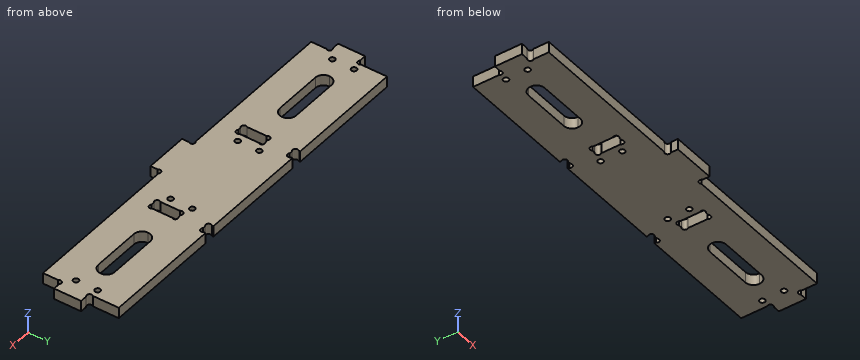
Autodesk Inventor part; units mm, degrees
ref_plane "YZ Plane" through (0, 0, 0) normal (1, 0, 0) x (0, 1, 0)
ref_plane "XZ Plane" through (0, 0, 0) normal (0, 1, 0) x (-1, 0, 0)
ref_plane "XY Plane" through (0, 0, 0) normal (0, 0, 1) x (1, 0, 0)
sketch "Sketch1" plane through (0, 0, 0) normal (0, 0, 1) x (1, 0, 0)
  line L0 (0, 0) -> (457.2, 0)
  line L1 (457.2, 0) -> (457.2, 101.6)
  line L2 (457.2, 101.6) -> (0, 101.6)
  line L3 (0, 101.6) -> (0, 0)
  line L4 (0, 101.6) -> (12.7, 101.6)
  line L5 (12.7, 101.6) -> (12.7, 66.675)
  line L6 (12.7, 66.675) -> (0, 66.675)
  line L7 (0, 66.675) -> (0, 101.6)
  line L8 (457.2, 101.6) -> (444.5, 101.6)
  line L9 (444.5, 101.6) -> (444.5, 66.675)
  line L10 (444.5, 66.675) -> (457.2, 66.675)
  line L11 (457.2, 66.675) -> (457.2, 101.6)
  line L12 (0, 0) -> (12.7, 0)
  line L13 (12.7, 0) -> (12.7, 34.925)
  line L14 (12.7, 34.925) -> (0, 34.925)
  line L15 (0, 34.925) -> (0, 0)
  line L16 (457.2, 0) -> (444.5, 0)
  line L17 (444.5, 0) -> (444.5, 34.925)
  line L18 (444.5, 34.925) -> (457.2, 34.925)
  line L19 (457.2, 34.925) -> (457.2, 0)
  line L20 (152.4, 101.6) -> (165.1, 101.6)
  line L21 (165.1, 101.6) -> (165.1, 95.25)
  line L22 (165.1, 95.25) -> (152.4, 95.25)
  line L23 (152.4, 95.25) -> (152.4, 101.6)
  line L24 (304.8, 101.6) -> (292.1, 101.6)
  line L25 (292.1, 101.6) -> (292.1, 95.25)
  line L26 (292.1, 95.25) -> (304.8, 95.25)
  line L27 (304.8, 95.25) -> (304.8, 101.6)
  line L28 (152.4, 66.675) -> (165.1, 66.675)
  line L29 (165.1, 66.675) -> (165.1, 34.925)
  line L30 (165.1, 34.925) -> (152.4, 34.925)
  line L31 (152.4, 34.925) -> (152.4, 66.675)
  line L32 (292.1, 66.675) -> (304.8, 66.675)
  line L33 (304.8, 66.675) -> (304.8, 34.925)
  line L34 (304.8, 34.925) -> (292.1, 34.925)
  line L35 (292.1, 34.925) -> (292.1, 66.675)
  line L36 (12.7, 0) -> (203.2, 0)
  line L37 (203.2, 0) -> (203.2, 12.7)
  line L38 (203.2, 12.7) -> (12.7, 12.7)
  line L39 (12.7, 12.7) -> (12.7, 0)
  line L40 (444.5, 0) -> (254, 0)
  line L41 (254, 0) -> (254, 12.7)
  line L42 (254, 12.7) -> (444.5, 12.7)
  line L43 (444.5, 12.7) -> (444.5, 0)
  point P0 (0, 66.675)
  point P1 (12.7, 12.7)
  point P2 (292.1, 101.6)
  point P3 (165.1, 101.6)
  dimension "d0" = 101.6
  dimension "d1" = 457.2
  dimension "d2" = 12.7
  dimension "d3" = 34.925
  dimension "d4" = 12.7
  dimension "d5" = 34.925
  dimension "d6" = 12.7
  dimension "d7" = 34.925
  dimension "d8" = 12.7
  dimension "d9" = 34.925
  dimension "d13" = 12.7
  dimension "d14" = 6.35
  dimension "d15" = 139.7
  dimension "d16" = 12.7
  dimension "d17" = 6.35
  dimension "d18" = 139.7
  dimension "d19" = 12.7
  dimension "d20" = 139.7
  dimension "d21" = 28.575
  dimension "d22" = 12.7
  dimension "d23" = 139.7
  dimension "d24" = 28.575
  dimension "d25" = 31.75
  dimension "d26" = 31.75
  dimension "d27" = 190.5
  dimension "d28" = 12.7
  dimension "d29" = 190.5
  dimension "d30" = 12.7
extrude "Extrusion1" add sketch "Sketch1" along normal blind 12.7 contours L3 L6 L5 L2 L23 L22 L21 L25 L26 L27 L9 L10 L1 L18 L17 L42 L41 L0 L37 L38 L13 L14
sketch "Sketch3" plane through (0, 0, 12.7) normal (0, 0, 1) x (1, 0, 0)
  line L0 (12.7, 101.6) -> (12.7, 66.675)
  line L1 (12.7, 66.675) -> (10.4549, 68.9201)
  circle A0 centre (10.4549, 68.9201) radius 3.175
  line L2 (12.7, 34.925) -> (12.7, 12.7)
  line L3 (12.7, 34.925) -> (10.4549, 32.6799)
  circle A1 centre (10.4549, 32.6799) radius 3.175
  line L4 (203.2, 12.7) -> (203.2, 0)
  line L5 (203.2, 12.7) -> (200.9549, 10.4549)
  circle A2 centre (200.9549, 10.4549) radius 3.175
  line L6 (254, 0) -> (254, 12.7)
  line L7 (254, 12.7) -> (256.2451, 10.4549)
  line L8 (254, 12.7) -> (444.5, 12.7)
  circle A3 centre (256.2451, 10.4549) radius 3.175
  line L9 (444.5, 34.925) -> (446.7451, 32.6799)
  line L10 (444.5, 34.925) -> (457.2, 34.925)
  circle A4 centre (446.7451, 32.6799) radius 3.175
  line L11 (457.2, 66.675) -> (444.5, 66.675)
  line L12 (444.5, 66.675) -> (446.7451, 68.9201)
  circle A5 centre (446.7451, 68.9201) radius 3.175
  line L13 (304.8, 34.925) -> (292.1, 34.925)
  line L14 (292.1, 34.925) -> (294.3451, 37.1701)
  line L15 (304.8, 34.925) -> (302.5549, 37.1701)
  line L16 (304.8, 66.675) -> (304.8, 34.925)
  line L17 (292.1, 66.675) -> (304.8, 66.675)
  line L18 (292.1, 66.675) -> (294.3451, 64.4299)
  line L19 (304.8, 66.675) -> (302.5549, 64.4299)
  line L20 (304.8, 95.25) -> (292.1, 95.25)
  line L21 (292.1, 95.25) -> (294.3451, 97.4951)
  line L22 (304.8, 95.25) -> (302.5549, 97.4951)
  line L23 (304.8, 101.6) -> (304.8, 95.25)
  line L24 (165.1, 34.925) -> (152.4, 34.925)
  line L25 (152.4, 34.925) -> (154.6451, 37.1701)
  line L26 (165.1, 66.675) -> (165.1, 34.925)
  line L27 (165.1, 34.925) -> (162.8549, 37.1701)
  line L28 (152.4, 66.675) -> (165.1, 66.675)
  line L29 (152.4, 66.675) -> (154.6451, 64.4299)
  line L30 (165.1, 66.675) -> (162.8549, 64.4299)
  line L31 (165.1, 95.25) -> (152.4, 95.25)
  line L32 (152.4, 95.25) -> (154.6451, 97.4951)
  line L33 (165.1, 95.25) -> (162.8549, 97.4951)
  line L34 (165.1, 101.6) -> (165.1, 95.25)
  circle A6 centre (154.6451, 97.4951) radius 3.175
  circle A7 centre (162.8549, 97.4951) radius 3.175
  circle A8 centre (154.6451, 64.4299) radius 3.175
  circle A9 centre (162.8549, 64.4299) radius 3.175
  circle A10 centre (162.8549, 37.1701) radius 3.175
  circle A11 centre (154.6451, 37.1701) radius 3.175
  circle A12 centre (294.3451, 37.1701) radius 3.175
  circle A13 centre (302.5549, 37.1701) radius 3.175
  circle A14 centre (294.3451, 64.4299) radius 3.175
  circle A15 centre (302.5549, 64.4299) radius 3.175
  circle A16 centre (294.3451, 97.4951) radius 3.175
  circle A17 centre (302.5549, 97.4951) radius 3.175
  point P0 (0, 0)
  dimension "d38" = 3.175
  dimension "d39" = 45
  dimension "d40" = 6.35
  dimension "d41" = 3.175
  dimension "d42" = 45
  dimension "d43" = 6.35
  dimension "d44" = 3.175
  dimension "d45" = 45
  dimension "d46" = 6.35
  dimension "d47" = 3.175
  dimension "d48" = 45
  dimension "d49" = 6.35
  dimension "d50" = 3.175
  dimension "d51" = 45
  dimension "d52" = 6.35
  dimension "d53" = 3.175
  dimension "d54" = 45
  dimension "d55" = 6.35
  dimension "d56" = 3.175
  dimension "d57" = 45
  dimension "d58" = 3.175
  dimension "d59" = 45
  dimension "d60" = 3.175
  dimension "d61" = 45
  dimension "d62" = 3.175
  dimension "d63" = 45
  dimension "d64" = 3.175
  dimension "d65" = 45
  dimension "d66" = 3.175
  dimension "d67" = 45
  dimension "d68" = 3.175
  dimension "d69" = 45
  dimension "d70" = 3.175
  dimension "d71" = 45
  dimension "d72" = 3.175
  dimension "d73" = 45
  dimension "d74" = 3.175
  dimension "d75" = 45
  dimension "d76" = 3.175
  dimension "d77" = 45
  dimension "d78" = 3.175
  dimension "d79" = 45
  dimension "d80" = 6.35
  dimension "d81" = 6.35
  dimension "d82" = 6.35
  dimension "d83" = 6.35
  dimension "d84" = 6.35
  dimension "d85" = 6.35
  dimension "d86" = 6.35
  dimension "d87" = 6.35
  dimension "d88" = 6.35
  dimension "d89" = 6.35
  dimension "d90" = 6.35
  dimension "d91" = 6.35
extrude "Extrusion3" cut sketch "Sketch3" against normal blind 25.4
sketch "Sketch6" plane through (0, 0, 12.7) normal (0, 0, 1) x (1, 0, 0)
  circle A0 centre (22.225, 69.85) radius 3.175
  line L0 (152.4, 101.6) -> (12.7, 101.6)
  line L1 (12.7, 101.6) -> (12.7, 71.1651)
  circle A1 centre (174.625, 69.85) radius 3.175
  line L2 (292.1, 101.6) -> (165.1, 101.6)
  line L3 (165.1, 62.1849) -> (165.1, 39.4151)
  circle A2 centre (282.575, 69.85) radius 3.175
  line L4 (292.1, 39.4151) -> (292.1, 62.1849)
  circle A3 centre (282.575, 44.45) radius 3.175
  circle A4 centre (174.625, 44.45) radius 3.175
  circle A5 centre (22.225, 44.45) radius 3.175
  circle A6 centre (434.975, 69.85) radius 3.175
  line L5 (444.5, 101.6) -> (304.8, 101.6)
  line L6 (444.5, 71.1651) -> (444.5, 101.6)
  circle A7 centre (434.975, 44.45) radius 3.175
  line L7 (444.5, 12.7) -> (444.5, 30.4349)
  point P0 (0, 0)
  dimension "d146" = 6.35
  dimension "d147" = 31.75
  dimension "d148" = 9.525
  dimension "d149" = 6.35
  dimension "d150" = 31.75
  dimension "d151" = 9.525
  dimension "d152" = 6.35
  dimension "d153" = 31.75
  dimension "d154" = 9.525
  dimension "d155" = 6.35
  dimension "d156" = 9.525
  dimension "d157" = 25.4
  dimension "d158" = 6.35
  dimension "d159" = 9.525
  dimension "d160" = 25.4
  dimension "d161" = 6.35
  dimension "d162" = 9.525
  dimension "d163" = 25.4
  dimension "d164" = 6.35
  dimension "d165" = 31.75
  dimension "d166" = 9.525
  dimension "d167" = 6.35
  dimension "d168" = 9.525
  dimension "d169" = 25.4
extrude "Extrusion5" cut sketch "Sketch6" against normal blind 12.7
sketch "Sketch7" plane through (0, 0, 12.7) normal (0, 0, 1) x (1, 0, 0)
  line L0 (44.45, 66.675) -> (120.65, 66.675)
  line L1 (120.65, 66.675) -> (120.65, 47.625)
  line L2 (120.65, 47.625) -> (44.45, 47.625)
  line L3 (44.45, 47.625) -> (44.45, 66.675)
  line L4 (12.7, 101.6) -> (12.7, 71.1651)
  line L5 (152.4, 101.6) -> (12.7, 101.6)
  line L6 (336.55, 66.675) -> (412.75, 66.675)
  line L7 (412.75, 66.675) -> (412.75, 47.625)
  line L8 (412.75, 47.625) -> (336.55, 47.625)
  line L9 (336.55, 47.625) -> (336.55, 66.675)
  line L10 (444.5, 101.6) -> (304.8, 101.6)
  line L11 (444.5, 12.7) -> (444.5, 30.4349)
  point P0 (0, 0)
  point P1 (82.55, 66.675)
  point P2 (44.45, 57.15)
  point P3 (412.75, 57.15)
  point P4 (374.65, 66.675)
  dimension "d172" = 19.05
  dimension "d173" = 76.2
  dimension "d174" = 69.85
  dimension "d175" = 44.45
  dimension "d176" = 76.2
  dimension "d177" = 19.05
  dimension "d178" = 44.45
  dimension "d179" = 69.85
extrude "Extrusion6" cut sketch "Sketch7" against normal blind 12.7
fillet "Fillet1" radius 9.525 8 edges at (44.45, 47.625, 6.35) (44.45, 66.675, 6.35) (120.65, 66.675, 6.35) (120.65, 47.625, 6.35) (336.55, 66.675, 6.35) (336.55, 47.625, 6.35) (412.75, 47.625, 6.35) (412.75, 66.675, 6.35)
properties part number "Inner Front Wall"
Model file for the job. Use its own axes, mm. Round coordinates to 2 decimals unless told otherwise and drop trailing zeros. Loops run counter-clockwise (first coordinate to the right, second up) from the corner with the lowest first, then second, coordinate; pieces in that order, holes last. Notation, with made-up numbers: (-11.75, 47.25) -> (-3.75, 47.25) arc R26 cw to (-3.75, 73.25) -> close; hole circle Ø4 at (9, -21). An arc over 180 degrees is marked (long way). Answer as CSV lines item,"result". Start each with the question number.
1) Slice it at A-A (x = 71). List the corners of the cut face in (y, z) (3 decimals).
2) Slice it at B-B (z = 7.5). State how many separate pieces and enclosed holes the cut face has, plus the area to 3 significant figures.
3) Slice it at D-D (x = 263). List the corners of the cut face in (y, z).
4) Slice it at C-C (y = 89). List the corners of the cut face in (x, z).
5) Probe line 1 along Y through (x, z) = (382, 1) (3 decimals); line 2 along X through (y, z) = (59, 7.5); line 3 along X through (y, z) = (96, 3). List the from-to ranges inside material, lowest first.
6) Pin check, flat tips, straight feed: P1, Ø6, axis at y = 84.5, z = 8.5, coming from the -X side; P2, Ø6.5, axis at x = 454.5, z = 9, coming from the +Y side (3 decimals); P3, Ø6.5, axis at x = 87.5, z = 6.5, coming from the -Y side. Stop position of each tip, or through.
Filled in:
1,outline,"(12.7, 0) -> (47.625, 0) -> (47.625, 12.7) -> (12.7, 12.7) -> close; (66.675, 0) -> (101.6, 0) -> (101.6, 12.7) -> (66.675, 12.7) -> close"
2,separate pieces,"1"
2,enclosed holes,"12"
2,area,"35,800 mm2"
3,outline,"(12.7, 0) -> (101.6, 0) -> (101.6, 12.7) -> (12.7, 12.7) -> close"
4,outline,"(12.7, 0) -> (444.5, 0) -> (444.5, 12.7) -> (12.7, 12.7) -> close"
5,line 1,"y = 12.7 to 47.625, 66.675 to 101.6"
5,line 2,"x = 0 to 44.63, 120.47 to 152.4, 165.1 to 292.1, 304.8 to 336.73, 412.57 to 457.2"
5,line 3,"x = 12.7 to 151.84, 165.66 to 291.54, 305.36 to 444.5"
6,P1,"stops at x = 12.7"
6,P2,"stops at y = 66.675"
6,P3,"stops at y = 12.7"
